from build123d import *

# Parameters (mm, degrees)
SKETCH1_R                                      = 340
SKETCH1_R_2                                    = 250
BOSS_EXTRUDE1_DEPTH                            = 12
BOSS_EXTRUDE2_DEPTH                            = 12
CIRPATTERN1_COUNT                              = 3
CUT_EXTRUDE1_DEPTH                             = 12
CIRPATTERN2_COUNT                              = 3
CUT_EXTRUDE2_DEPTH                             = 12
SKETCH8_R                                      = 10
CUT_EXTRUDE3_DEPTH                             = 12
SKETCH9_W                                      = 60
SKETCH9_H                                      = 20
CUT_EXTRUDE4_DEPTH                             = 12
FILLET1_R                                      = 5
CSK_FOR_M4_FLAT_HEAD_MACHINE_SCREW_D           = 4.5
CSK_FOR_M4_FLAT_HEAD_MACHINE_SCREW_CSINK_D     = 9.4
CSK_FOR_M4_FLAT_HEAD_MACHINE_SCREW_CSINK_ANGLE = 90


with BuildPart() as part:
    # Sketch1 → Boss-Extrude1 (new body)
    with BuildSketch(Plane(origin=(0, 0, 0), x_dir=(1, 0, 0), z_dir=(0, 1, 0))):
        Circle(SKETCH1_R)
        Circle(SKETCH1_R_2, mode=Mode.SUBTRACT)
    extrude(amount=BOSS_EXTRUDE1_DEPTH)

    # Sketch2 → Boss-Extrude2 (add)
    with BuildSketch(Plane.XZ):
        with BuildLine():
            Line((351.85982974, 133.864335114), (319.827534924, 115.37048108))
            ThreePointArc((319.827534924, 115.37048108), (294.448637287, 170), (259.827534924, 219.293529534))
            Line((259.827534924, 219.293529534), (291.85982974, 237.787383569))
            ThreePointArc((291.85982974, 237.787383569), (298.796843602, 238.937734879), (304.776091866, 235.237186318))
            ThreePointArc((304.776091866, 235.237186318), (333.419780457, 192.5), (356.109425199, 146.325244863))
            ThreePointArc((356.109425199, 146.325244863), (356.324570129, 139.29678969), (351.85982974, 133.864335114))
        make_face()
        with BuildLine():
            ThreePointArc((298.990496165, 209.355399268), (316.099272381, 182.5), (330.802342268, 154.255665535))
            ThreePointArc((330.802342268, 154.255665535), (328.383894642, 147.611035291), (321.739264398, 150.029482918))
            ThreePointArc((321.739264398, 150.029482918), (307.439018343, 177.5), (290.798975723, 203.619634905))
            ThreePointArc((290.798975723, 203.619634905), (292.026853762, 210.583277308), (298.990496165, 209.355399268))
        make_face(mode=Mode.SUBTRACT)
    boss_extrude2 = extrude(amount=-BOSS_EXTRUDE2_DEPTH)

    # CirPattern1: Boss-Extrude2 ×3 about axis
    cirpattern1_axis = Axis((0, 0, 0), (0, 1, 0))
    for i in range(1, CIRPATTERN1_COUNT):
        add(boss_extrude2.rotate(cirpattern1_axis, i * 360 / CIRPATTERN1_COUNT))

    # Sketch6 → Cut-Extrude1 (cut)
    with BuildSketch(Plane(origin=(0, 12, 0), x_dir=(1, 0, 0), z_dir=(0, 1, 0))):
        with BuildLine():
            Line((234.923155199, -85.505035825), (248.308329747, -90.37684094))
            ThreePointArc((248.308329747, -90.37684094), (264.279563148, -89.37703061), (274.405240734, -76.985478225))
            ThreePointArc((274.405240734, -76.985478225), (246.817240074, 142.500000006), (70.531240487, 276.134648524))
            ThreePointArc((70.531240487, 276.134648524), (54.737002537, 273.561330696), (45.885524691, 260.229742005))
            Line((45.885524691, 260.229742005), (43.412044408, 246.201938255))
            ThreePointArc((43.412044408, 246.201938255), (216.506350942, 125.000000007), (234.923155199, -85.505035825))
        make_face()
    cut_extrude1 = extrude(amount=-CUT_EXTRUDE1_DEPTH, mode=Mode.SUBTRACT)

    # CirPattern2: Cut-Extrude1 ×3 about axis
    cirpattern2_axis = Axis((0, 0, 0), (0, 1, 0))
    for i in range(1, CIRPATTERN2_COUNT):
        add(cut_extrude1.rotate(cirpattern2_axis, i * 360 / CIRPATTERN2_COUNT), mode=Mode.SUBTRACT)

    # Sketch7 → Cut-Extrude2 (cut)
    with BuildSketch(Plane.XZ):
        with BuildLine():
            Line((-81.853527719, 330), (81.853527719, 330))
            ThreePointArc((81.853527719, 330), (0, 340), (-81.853527719, 330))
        make_face()
    extrude(amount=-CUT_EXTRUDE2_DEPTH, mode=Mode.SUBTRACT)

    # Sketch8 → Cut-Extrude3 (cut)
    with BuildSketch(Plane(origin=(0, 12, 0), x_dir=(1, 0, 0), z_dir=(0, 1, 0))):
        with Locations((0, 290)):
            Circle(SKETCH8_R)
        with Locations((251.147367097, -145)):
            Circle(SKETCH8_R)
        with Locations((-251.147367097, -145)):
            Circle(SKETCH8_R)
    extrude(amount=-CUT_EXTRUDE3_DEPTH, mode=Mode.SUBTRACT)

    # Sketch9 → Cut-Extrude4 (cut)
    with BuildSketch(Plane(origin=(0, 12, 0), x_dir=(1, 0, 0), z_dir=(0, 1, 0))):
        with Locations((0, -320)):
            Rectangle(SKETCH9_W, SKETCH9_H)
    extrude(amount=-CUT_EXTRUDE4_DEPTH, mode=Mode.SUBTRACT)

    # Fillet1
    fillet1_edges = [part.edges().sort_by_distance(p)[0] for p in [
        (30, 6, 330),
        (-30, 6, 330),
        (-30, 6, 310),
        (30, 6, 310),
    ]]
    fillet(fillet1_edges, radius=FILLET1_R)

    # CSK for M4 Flat Head Machine Screw (through all)
    with Locations(Plane(origin=(0, 48, 0), x_dir=(1, 0, 0), z_dir=(0, 1, 0))):
        with Locations((80.233903982, 299.43700615), (219.203102168, 219.203102168), (299.43700615, 80.233903982), (299.43700615, -80.233903982), (219.203102168, -219.203102168), (80.233903982, -299.43700615), (-80.233903982, -299.43700615), (-219.203102168, -219.203102168), (-299.43700615, -80.233903982), (-299.43700615, 80.233903982), (-219.203102168, 219.203102168), (-80.233903982, 299.43700615), (0, 0)):
            CounterSinkHole(CSK_FOR_M4_FLAT_HEAD_MACHINE_SCREW_D / 2, CSK_FOR_M4_FLAT_HEAD_MACHINE_SCREW_CSINK_D / 2, counter_sink_angle=CSK_FOR_M4_FLAT_HEAD_MACHINE_SCREW_CSINK_ANGLE)


solid = part.part
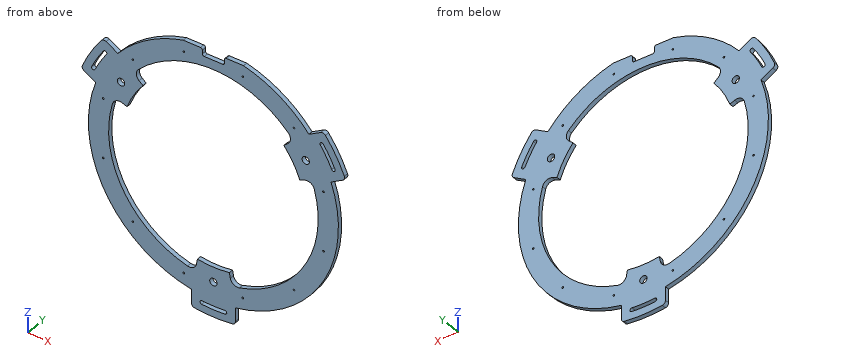
Build history of the part. All positions in model axes, mm. Round coordinates to 2 decimals unless told otherwise and drop trailing zeros. Loops run counter-clockwise (first coordinate to the right, second up) from the corner with the lowest first, then second, coordinate; pieces in that order, holes last. Notation, with made-up numbers: (82, 41) -> (131, 41) arc R11 ccw to (131, 47) -> close; hole circle Ø5 at (-30, 30.25). An arc over 180 degrees is marked (long way). Answer in a Markdown table with one row per item.
Item 1: Saw through at C-C (z = -32.5). Write the cut outline in (x, y).
Answers below:
| item | result |
|---|---|
| outline | (-338.44, 0) -> (-283.14, 0) -> (-283.14, 12) -> (-338.44, 12) -> close; (283.14, 0) -> (338.44, 0) -> (338.44, 12) -> (283.14, 12) -> close |
Item 2: Saw through at D-D (y = 8.5). State how many separate pieces and enclosed holes the cut face has, and give its area (3 significant figures).
Answers below:
| item | result |
|---|---|
| separate pieces | 1 |
| enclosed holes | 19 |
| area | 129,000 mm² |
Item 3: Saw through at A-A (x = 0). Write the cut outline in (y, z).
Answers below:
| item | result |
|---|---|
| outline | (0, -385) -> (12, -385) -> (12, -365) -> (0, -365) -> close; (0, -355) -> (12, -355) -> (12, -300) -> (0, -300) -> close; (0, -280) -> (12, -280) -> (12, -250) -> (0, -250) -> close; (0, 285) -> (12, 285) -> (12, 310) -> (0, 310) -> close |
Item 4: Saw through at B-B (x = -163.5). Write the cut outline in (y, z), and give its area (3 significant figures).
Answers below:
| item | result |
|---|---|
| outline | (0, -298.11) -> (12, -298.11) -> (12, -233.44) -> (0, -233.44) -> close; (0, 233.44) -> (12, 233.44) -> (12, 298.11) -> (0, 298.11) -> close |
| area | 1,550 mm² |
Item 5: Drill centre lines: L1, parallel to X at y = 2.75, z = 201; L2, parallel to Z at x = -198, y = 8.25; L3, parallel to Z at x = -17.5, y = 1. Where is each one in solid material? Low to high. Write a range as [from, to].
Answers below:
| item | result |
|---|---|
| L1 | x = [-328.37, -304.67], [-292.62, -202.05], [202.05, 292.62], [304.67, 328.37] |
| L2 | z = [-276.4, -204.99], [152.63, 166.14], [204.99, 276.4] |
| L3 | z = [-384.6, -364.58], [-354.57, -249.39], [284.46, 310] |
Item 6: Pin check, flat tips, straight feed: pin 1 (16 mm diameter, centred on x = 251.15, z = 145, fed in from +Y); pin 2 (2 mm diameter, centred on y = 5.5, z = -244.5, fed in from -X); pin 3 (1.5 mm diameter, centred on y = 3, z = -154, fed in from +X); pin 4 (6 mm diameter, centred on x = 12, y = 4, fed in from +Z). Stop position of each tip, or through.
Answers below:
| item | result |
|---|---|
| pin 1 | passes through |
| pin 2 | stops at x = -237.29 |
| pin 3 | stops at x = 303.5 |
| pin 4 | stops at z = 310 |
